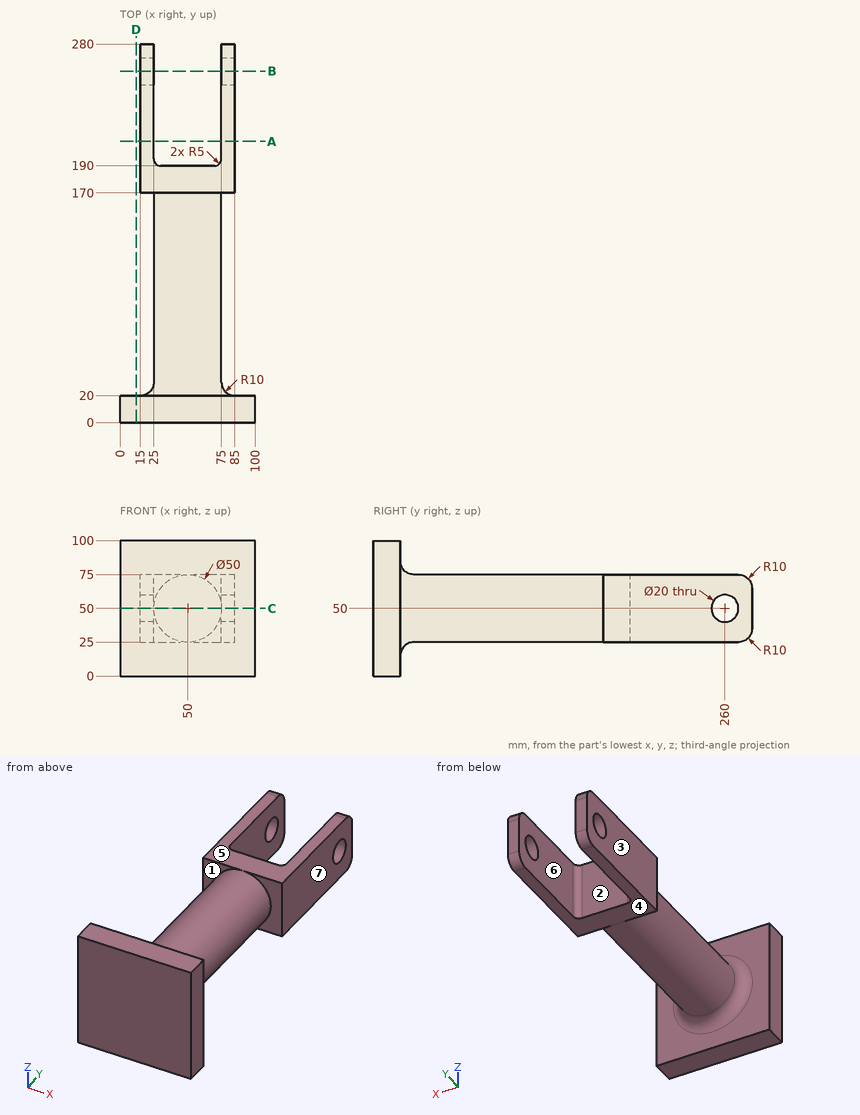
Design review of the part shown in the three views and the two pictorial views. Dimensions are in mm from the part's minimum x, y and z. A direction names the side the tool comes from. Give positions to 0.01 mm unless a question says otherwise; leave off trailing zeros. Order: outer loops, then holes, each group sorted by start corner. A loop starts at its lowest first (then second) coordinate and runs counter-clockwise, first axis right, second up. Notation, with made-up numbers: (17, 81) -> (37, 81) arc R19 ccw to (37, 117) -> close; hole circle Ø3 at (44.5, 49). An arc over 180 degrees is marked (long way). Write each question's results on one line, items separated by ' | '. Start each with the question number.
Q1. Mouldability with a two-part tool opening along X and no side actions: class the marked faces 1, 2 and 3 as +X half, -X half, draft (parallel to the pull), parting line (faces both ways), or undercut.
Q2. Add section B-B on y = 260. Give the boundary of the cut face in (x, z).
Q3. Machinability: for the marked faces 4, 5, 6 and 7, which of the approach directions +Z, -Z, +X, -X, +Y, -Y give a long, thin tool a straight path to every point of the face, cutting with its end or side? Answer none if there is none.
Q4. For pin 1 (6 mm diameter, centred on x = 64, y = 131.5, fed in from +Z); pin 2 (5 mm diameter, centred on y = 39.5, z = 31, fed in from -X); pin 3 (3 mm diameter, centred on y = 162.5, z = 41, fed in from -X); pin 4 (17.5 mm diameter, centred on x = 30.5, z = 49, fed in from -Y), all flat-tipped, find the tip position at first contact; note any pin that passes through.
Q5. Wall thickness on L1, parallel to Y at x = 81, z = 50; L2, parallel to X at y = 207.5, z = 31.5; L3, parallel to Y at x = 19.5, z = 50: over which ranges is each line inside the solid? List them lowest first. Write a range as from..to.
Q6. Add section A-A on y = 208. Give the boundary of the cut face in (x, z).
Q7. Add section C-C on z = 50. Give the boundary of the cut face in (x, y).
Q8. Add section D-D on x = 12. Give the boundary of the cut face in (y, z), and give its area (3 significant figures).
Found:
1) face 1: draft | face 2: undercut | face 3: -X half
2) outline: (15, 25) -> (25, 25) -> (25, 40) -> (15, 40) -> close; (15, 60) -> (25, 60) -> (25, 75) -> (15, 75) -> close; (75, 25) -> (85, 25) -> (85, 40) -> (75, 40) -> close; (75, 60) -> (85, 60) -> (85, 75) -> (75, 75) -> close
3) face 4: -Z, +X, -X, +Y | face 5: +Z, +X, -X, +Y | face 6: +Z, -Z, +Y | face 7: +Z, -Z, +X, +Y
4) pin 1: stops at z = 72.45 | pin 2: stops at x = 31.22 | pin 3: stops at x = 26.15 | pin 4: stops at y = 0
5) L1: y = 0..20.83, 170..250, 270..280 | L2: x = 15..25, 75..85 | L3: y = 0..21.07, 170..250, 270..280
6) outline: (15, 25) -> (25, 25) -> (25, 75) -> (15, 75) -> close; (75, 25) -> (85, 25) -> (85, 75) -> (75, 75) -> close
7) outline: (0, 0) -> (100, 0) -> (100, 20) -> (85, 20) arc R10 cw to (75, 30) -> (75, 170) -> (85, 170) -> (85, 250) -> (75, 250) -> (75, 195) arc R5 cw to (70, 190) -> (30, 190) arc R5 cw to (25, 195) -> (25, 250) -> (15, 250) -> (15, 170) -> (25, 170) -> (25, 30) arc R10 cw to (15, 20) -> (0, 20) -> close; (15, 270) -> (25, 270) -> (25, 280) -> (15, 280) -> close; (75, 270) -> (85, 270) -> (85, 280) -> (75, 280) -> close
8) outline: (0, 0) -> (20, 0) -> (20, 100) -> (0, 100) -> close | area: 2,000 mm2
